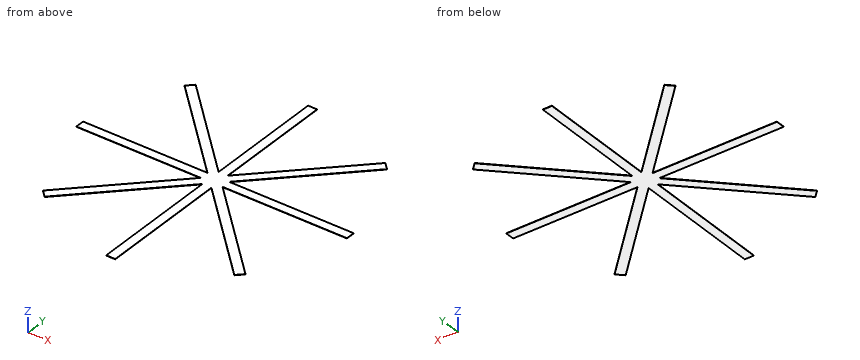
```python
from build123d import *

# Parameters (mm, degrees)
F1_DEPTH = 0.2


# Not quite as in the source:
# - a feature names something its author has since deleted; it is built from what else it names


with BuildPart() as f1:
    # F0 (on Top) → F1 (new body)
    with BuildSketch(Plane.XY):
        Polygon((3, 87.0174653775), (-3, 87.0174653775), (-3, 7.2426406871), (-3, 3), (3, 3), (3, 7.2426406871), align=None)
        Polygon((-7.2426406871, 3), (-3, 7.2426406871), (-63.1040764009, 67.346717088), (-67.346717088, 63.1040764009), align=None)
        Polygon((-3, 3), (-3, 7.2426406871), (-7.2426406871, 3), align=None)
        Polygon((7.2426406871, 3), (3, 7.2426406871), (3, 3), align=None)
        Polygon((63.1040764009, 67.346717088), (3, 7.2426406871), (7.2426406871, 3), (67.346717088, 63.1040764009), align=None)
        Polygon((3, 3), (-3, 3), (-3, 0), (0, 0), (3, 0), align=None)
        Polygon((-3, 0), (-3, 3), (-7.2426406871, 3), (-90, 3), (-90, -3), (-7.2426406871, -3), (-3, -3), align=None)
        Polygon((7.2426406871, 3), (3, 3), (3, 0), (3, -3), (7.2426406871, -3), (90, -3), (90, 3), align=None)
        Polygon((0, 0), (-3, 0), (-3, -3), (3, -3), (3, 0), align=None)
        Polygon((3, -3), (-3, -3), (-3, -7.2426406871), (-3, -92.9825346225), (3, -92.9825346225), (3, -7.2426406871), align=None)
        Polygon((-3, -7.2426406871), (-3, -3), (-7.2426406871, -3), align=None)
        Polygon((7.2426406871, -3), (3, -3), (3, -7.2426406871), align=None)
        Polygon((-63.1040764009, -67.346717088), (-3, -7.2426406871), (-7.2426406871, -3), (-67.346717088, -63.1040764009), align=None)
        Polygon((7.2426406871, -3), (3, -7.2426406871), (63.1040764009, -67.346717088), (67.346717088, -63.1040764009), align=None)
    extrude(amount=F1_DEPTH)


solid = f1.part
```
The model under review builds one solid part; all positions refer to its coordinate system, in mm. Round coordinates to 2 decimals unless told otherwise and drop trailing zeros. Loops run counter-clockwise (first coordinate to the right, second up) from the corner with the lowest first, then second, coordinate; pieces in that order, holes last. Notation, with made-up numbers: (84, 79.5) -> (119, 79.5) arc R12 cw to (119, 97.5) -> close; hole circle Ø10 at (68, 43.25). An arc over 180 degrees is marked (long way). Answer in a Markdown table with one row per item.
1) Consider section A-A, the plane z = 0.15. Write out the cut boundary in (x, y), plus the area to 3 significant figures.
Taken from the geometry:
| item | result |
|---|---|
| outline | (-90, -3) -> (-7.24, -3) -> (-67.35, -63.1) -> (-63.1, -67.35) -> (-3, -7.24) -> (-3, -92.98) -> (3, -92.98) -> (3, -7.24) -> (63.1, -67.35) -> (67.35, -63.1) -> (7.24, -3) -> (90, -3) -> (90, 3) -> (7.24, 3) -> (67.35, 63.1) -> (63.1, 67.35) -> (3, 7.24) -> (3, 87.02) -> (-3, 87.02) -> (-3, 7.24) -> (-63.1, 67.35) -> (-67.35, 63.1) -> (-7.24, 3) -> (-90, 3) -> close |
| area | 4,200 mm² |
2) Consider section B-B, the plane x = 45. Write out the cut boundary in (y, z).
Taken from the geometry:
| item | result |
|---|---|
| outline | (-49.24, 0) -> (-40.76, 0) -> (-40.76, 0.2) -> (-49.24, 0.2) -> close; (-3, 0) -> (3, 0) -> (3, 0.2) -> (-3, 0.2) -> close; (40.76, 0) -> (49.24, 0) -> (49.24, 0.2) -> (40.76, 0.2) -> close |
3) Wall thickness on line 1 along Y through (x, z) = (-26.5, 0.1); line 2 along X through (y, z) = (45, 0.1); line 3 along X through (y, z) = (-9, 0.15): over which ranges is each line inside the solid? List them lowest first.
Taken from the geometry:
| item | result |
|---|---|
| line 1 | y = -30.74 to -22.26, -3 to 3, 22.26 to 30.74 |
| line 2 | x = -49.24 to -40.76, -3 to 3, 40.76 to 49.24 |
| line 3 | x = -13.24 to -4.76, -3 to 3, 4.76 to 13.24 |
4) Consider section C-C, the plane y = -41. Write out the cut boundary in (x, z), plus the area to 3 significant figures.
Taken from the geometry:
| item | result |
|---|---|
| outline | (-45.24, 0) -> (-36.76, 0) -> (-36.76, 0.2) -> (-45.24, 0.2) -> close; (-3, 0) -> (3, 0) -> (3, 0.2) -> (-3, 0.2) -> close; (36.76, 0) -> (45.24, 0) -> (45.24, 0.2) -> (36.76, 0.2) -> close |
| area | 4.59 mm² |
5) Consider section D-D, the plane x = -75. Write out the cut boundary in (y, z).
Taken from the geometry:
| item | result |
|---|---|
| outline | (-3, 0) -> (3, 0) -> (3, 0.2) -> (-3, 0.2) -> close |
